Here's how the part is built. I have some questions about the finished solid (model axes, mm). A direction names the side the tool comes from. Round coordinates to 2 decimals unless told otherwise and drop trailing zeros. Order: outer loops, then holes, each group sorted by start corner. A loop starts at its lowest first (then second) coordinate and runs counter-clockwise, first axis right, second up. Notation, with made-up numbers: M -26,-29 L 1,-29 A25 cw 1,-8 Z; hole C 0,4 d8. An arc over 180 degrees is marked long. Write item = value, one per line. Start each with the question number.
Item 1: I want a section at A-A, the plane x = 7.5. List the corners of the cut face in (y, z) for me, plus the area to 3 significant figures.
Item 2: I'm going to push flat-ended pins straight in: P1, Ø2, axis at x = -24.5, y = 20, coming from the +Z side; P2, Ø2.5, axis at x = 7.5, y = -14.5, coming from the -Z side; P3, Ø2, axis at x = -6, y = -10.5, coming from the +Z side. Where does each tip first touch, or does it pass through?
Item 3: We'd pull the mould along X, two halves only. Please class faces 3 (the face through (-30, 0, 1)), 4 (the face through (25.03, -20.52, 0.62)), 5 (the face through (0, -24, 9)), 6 (the face through (9, -14.43, -8.01)): pulls with the +X half, pulls with the -X half, needs draft (parallel to the pull), parting line crosses it, or undercut.
Item 4: For faces 1 (the face through (-11.25, 22, 2)), 2 (the face through (-10, 22, -6)), which set-ups out of +Z, -Z, +X, -X, +Y, -Y let a thin tool reach every point of the face, with its end or its side?
Item 5: I want a section at C-C, the plane x = 24.5. List the corners of the cut face in (y, z) for me.
Item 6: Please list where these lines run through material, in increasing order: L1, parallel to Y at x = -24.5, z = 2.5; L2, parallel to Y at x = 7.5, z = -8.1; L3, parallel to Y at x = 1.5, z = 5.
Item 7: I want a section at B-B, the plane y = 0. List the corners of the cut face in (x, z) for me, plus the area to 3 significant figures.
Item 8: I want a section at D-D, the plane y = 14.5. List the corners of the cut face in (x, z) for me.
```python
from build123d import *

# Parameters (mm, degrees)
SKETCH2_W            = 60
SKETCH2_H            = 50
BOSS_EXTRUDE1_DEPTH  = 9
SHELL1_T             = -2
SKETCH6_R            = 11.75
SKETCH6_R_2          = 1.5
CUT_EXTRUDE3_DEPTH   = 18
SKETCH8_R            = 3.6
BOSS_EXTRUDE7_DEPTH  = 16
SKETCH10_R           = 3.6
BOSS_EXTRUDE8_DEPTH  = 16
SKETCH11_R           = 1.15
CUT_EXTRUDE4_DEPTH   = 17
SKETCH12_W           = 2
SKETCH12_H           = 2
BOSS_EXTRUDE13_DEPTH = 15
FILLET3_R            = 1


with BuildPart() as part:
    # Sketch2 → Boss-Extrude1 (new, symmetric)
    with BuildSketch(Plane.XY):
        Rectangle(SKETCH2_W, SKETCH2_H)
    extrude(amount=BOSS_EXTRUDE1_DEPTH, both=True)

    # Shell1
    shell1_openings = [part.faces().sort_by_distance(p)[0] for p in [
        (0, 0, 9),
    ]]
    offset(amount=SHELL1_T, openings=shell1_openings, kind=Kind.INTERSECTION)

    # Sketch6 → Cut-Extrude3 (cut)
    with BuildSketch(Plane(origin=(0, 0, -9), x_dir=(-1, 0, 0), z_dir=(0, 0, -1))):
        with Locations((-7.5, 0)):
            Circle(SKETCH6_R)
        with Locations((-7.5, 14.5)):
            Circle(SKETCH6_R_2)
        with Locations((-7.5, -14.5)):
            Circle(SKETCH6_R_2)
    extrude(amount=-CUT_EXTRUDE3_DEPTH, mode=Mode.SUBTRACT)

    # Sketch8 → Boss-Extrude7 (add, through all)
    with BuildSketch(Plane.XY.offset(-7)):
        with Locations((-24.5, 20)):
            Circle(SKETCH8_R)
    extrude(amount=BOSS_EXTRUDE7_DEPTH)

    # Sketch10 → Boss-Extrude8 (add, through all)
    with BuildSketch(Plane.XY.offset(-7)):
        with Locations((24.5, -19.5)):
            Circle(SKETCH10_R)
        with Locations((24.5, 19.5)):
            Circle(SKETCH10_R)
        with Locations((-24.5, -19.5)):
            Circle(SKETCH10_R)
    extrude(amount=BOSS_EXTRUDE8_DEPTH)

    # Sketch11 → Cut-Extrude4 (cut)
    with BuildSketch(Plane.XY.offset(9)):
        with Locations((-24.5, 20)):
            Circle(SKETCH11_R)
        with Locations((24.5, 19.5)):
            Circle(SKETCH11_R)
        with Locations((24.5, -19.5)):
            Circle(SKETCH11_R)
        with Locations((-24.5, -19.5)):
            Circle(SKETCH11_R)
    extrude(amount=-CUT_EXTRUDE4_DEPTH, mode=Mode.SUBTRACT)

    # Sketch12 → Boss-Extrude13 (add)
    with BuildSketch(Plane.XY.offset(9)):
        with Locations((-10.25, -22)):
            Rectangle(SKETCH12_W, SKETCH12_H)
        with Locations((-14.45, -22)):
            Rectangle(SKETCH12_W, SKETCH12_H)
        with Locations((-14.45, 22)):
            Rectangle(SKETCH12_W, SKETCH12_H)
        with Locations((-10.25, 22)):
            Rectangle(SKETCH12_W, SKETCH12_H)
    extrude(amount=-BOSS_EXTRUDE13_DEPTH)

    # Fillet3
    fillet3_edges = [part.edges().sort_by_distance(p)[0] for p in [
        (0, -25, -9),
        (-30, 0, -9),
        (0, 25, -9),
        (30, 0, -9),
        (30, -25, 0),
        (-30, -25, 0),
        (-30, 25, 0),
        (30, 25, 0),
    ]]
    fillet(fillet3_edges, radius=FILLET3_R)


solid = part.part
```
Filled in:
q1.outline = M -25,-8 A1 ccw -24,-9 L -16,-9 L -16,-7 L -23,-7 L -23,9 L -25,9 Z; M -13,-9 L -11.75,-9 L -11.75,-7 L -13,-7 Z; M 11.75,-9 L 13,-9 L 13,-7 L 11.75,-7 Z; M 16,-9 L 24,-9 A1 ccw 25,-8 L 25,9 L 23,9 L 23,-7 L 16,-7 Z
q1.area = 105 mm^2
q2.P1 = -8
q2.P2 = through
q2.P3 = -7
q3.face_3 = pulls with the -X half
q3.face_4 = undercut
q3.face_5 = needs draft
q3.face_6 = undercut
q4.face_1 = +Z
q4.face_2 = none
q5.outline = M -25,-8 A1 ccw -24,-9 L 24,-9 A1 ccw 25,-8 L 25,9 L 20.65,9 L 20.65,-8 L 18.35,-8 L 18.35,9 L 15.9,9 L 15.9,-7 L -15.9,-7 L -15.9,9 L -18.35,9 L -18.35,-8 L -20.65,-8 L -20.65,9 L -25,9 Z
q6.L1 = -25 to -20.65, -18.35 to -15.9, 16.4 to 18.85, 21.15 to 25
q6.L2 = -24.99 to -16, -13 to -11.75, 11.75 to 13, 16 to 24.99
q6.L3 = -25 to -23, 23 to 25
q7.outline = M -30,-8 A1 ccw -29,-9 L -4.25,-9 L -4.25,-7 L -28,-7 L -28,9 L -30,9 Z; M 19.25,-9 L 29,-9 A1 ccw 30,-8 L 30,9 L 28,9 L 28,-7 L 19.25,-7 Z
q7.area = 137 mm^2
q8.outline = M -30,-8 A1 ccw -29,-9 L 6,-9 L 6,-7 L -28,-7 L -28,9 L -30,9 Z; M 9,-9 L 29,-9 A1 ccw 30,-8 L 30,9 L 28,9 L 28,-7 L 9,-7 Z
